```python
from build123d import *


with BuildPart() as part:
    # Эскиз1 → Повернуть1 (revolve)
    with BuildSketch(Plane.XY, mode=Mode.PRIVATE) as revolve_1_sk:
        with BuildLine():
            Line((0, 34.5), (0, 37.5))
            Line((0, 37.5), (10, 37.5))
            Line((10, 37.5), (10, 33.5))
            ThreePointArc((10, 33.5), (10.292893219, 32.792893219), (11, 32.5))
            Line((11, 32.5), (17, 32.5))
            ThreePointArc((17, 32.5), (17.707106781, 32.792893219), (18, 33.5))
            Line((18, 33.5), (18, 37.5))
            Line((18, 37.5), (28, 37.5))
            Line((28, 37.5), (28, 24))
            Line((28, 24), (39, 24))
            Line((39, 24), (40, 23))
            Line((40, 23), (40, 16))
            Line((40, 16), (39, 15))
            Line((39, 15), (23, 15))
            Line((23, 15), (23, 15.5))
            Line((23, 15.5), (20, 15.5))
            Line((20, 15.5), (20, 0))
            Line((20, 0), (2, 0))
            Line((2, 0), (2, 34.5))
            Line((2, 34.5), (0, 34.5))
        make_face()
    revolve(revolve_1_sk.sketch.rotate(Axis((2, 0, 0), (1, 0, 0)), 180), axis=Axis((2, 0, 0), (1, 0, 0)))


solid = part.part
```
Here's how the part is built. I have some questions about the finished solid (model axes, mm). A direction names the side the tool comes from. Give positions to 0.01 mm unless a question says otherwise; leave off trailing zeros. Loops run counter-clockwise (first coordinate to the right, second up) from the corner with the lowest first, then second, coordinate; pieces in that order, holes last. Notation, with made-up numbers: M 57,-30 L 111,-30 A27 cw 111,-3 Z; hole C 24.25,56 d2. An arc over 180 degrees is marked long. Return JSON: item names as keys, results as strings.
Item 1: Imagine slicing it at C-C on x = 4. List the corners of the cut face in (y, z) for me.
A:
{"outline": "C 0,0 d75"}
Item 2: Imagine slicing it at B-B on x = 16. List the corners of the cut face in (y, z) for me, then the cut area to 3 significant figures.
A:
{"outline": "C 0,0 d65", "area": "3,320 mm^2"}
Item 3: On a 3-axis mill with a long thin cutter (end or side, diameter ignored), from which of +Z, -Z, +X, -X, +Y, -Y can I reach the whole of each face in a straight line? I mean faces 1 (the cylindrical face through (30.89, -8.06, -12.65)), 2 (the cylindrical face through (0.986, 34.467, -1.517)), 3 (the flat face through (23, -8, -13)), 4 (the flat face through (0, 33, 11)), 5 (the cylindrical face through (23.07, -17.3, 33.27)). Say none if no direction works.
A:
{"face 1": "+X", "face 2": "-X", "face 3": "none", "face 4": "+Z, -Z, -X, +Y, -Y", "face 5": "+X, -X"}
Item 4: Please list where these lines run through material, in increasing order: line 1 (Z direction, x = 32, y = 0); line 2 (X direction, y = 31, z = 14); line 3 (Z direction, x = 20.75, y = 0).
A:
{"line 1": "z = -24 to -15, 15 to 24", "line 2": "x = 2 to 10, 18 to 28", "line 3": "z = -37.5 to -15.5, 15.5 to 37.5"}
Item 5: I'm going to push flat-ended pins straight in: pin 1 Ø2 at (y, z) = (-27.5, -5) entering from +X; pin 2 Ø1.5 at (x, z) = (20.5, 16) entering from +Y; pin 3 Ø6 at (x, y) = (7, -17) entering from +Z. Where does each tip first touch, or does it pass through?
A:
{"pin 1": "stops at x = 28", "pin 2": "stops at y = 34.26", "pin 3": "stops at z = 34.79"}
Item 6: Imagine slicing it at A-A on x = 27. List the corners of the cut face in (y, z) for me.
A:
{"outline": "C 0,0 d75; hole C 0,0 d30"}
Item 7: Thinking about a two-plate mould opening in Y: for faces 6 (the cylindrical face through (14.04, -31, -9.76)), 7 (the flat face through (2, 0, 0)), 8 (the flat face through (20, 0, 0)), 9 (the flat face through (28, 0.5, 24.5)), which applies, released by +Y, released by -Y, zero draft, split by the parting line, or undercut?
A:
{"face 6": "split by the parting line", "face 7": "undercut", "face 8": "undercut", "face 9": "zero draft"}
